```python
from build123d import *

# Parameters (mm, degrees)
SKETCH_19_R           = 3.4
MEMBER_4060_A_1_DEPTH = 800
SKETCH_14_R           = 3
CUT_EXTRUDE_1_DEPTH   = 10


with BuildPart() as part:
    # 草图19 → Member 4060-a _1 (new body)
    with BuildSketch(Plane.YZ):
        with BuildLine():
            Line((10.25, 16.5), (10.25, 12.765240679))
            Line((10.25, 12.765240679), (6.149583391, 8.63609737))
            ThreePointArc((6.149583391, 8.63609737), (5.17375715, 7.980369349), (4.020871182, 7.75))
            Line((4.020871182, 7.75), (-4.020871182, 7.75))
            ThreePointArc((-4.020871182, 7.75), (-5.17375715, 7.980369349), (-6.149583391, 8.63609737))
            Line((-6.149583391, 8.63609737), (-10.25, 12.765240679))
            Line((-10.25, 12.765240679), (-10.25, 16.5))
            ThreePointArc((-10.25, 16.5), (-9.957106781, 17.207106781), (-9.25, 17.5))
            Line((-9.25, 17.5), (-8, 17.5))
            ThreePointArc((-8, 17.5), (-7.292893219, 17.207106781), (-7, 16.5))
            Line((-7, 16.5), (-7, 15.5))
            Line((-7, 15.5), (-4.1, 15.5))
            Line((-4.1, 15.5), (-4.1, 19))
            Line((-4.1, 19), (-5.1, 19))
            Line((-5.1, 19), (-5.1, 20))
            Line((-5.1, 20), (-27.5, 20))
            ThreePointArc((-27.5, 20), (-29.267766953, 19.267766953), (-30, 17.5))
            Line((-30, 17.5), (-30, 5.1))
            Line((-30, 5.1), (-29, 5.1))
            Line((-29, 5.1), (-29, 4.1))
            Line((-29, 4.1), (-25.5, 4.1))
            Line((-25.5, 4.1), (-25.5, 7))
            Line((-25.5, 7), (-26.5, 7))
            ThreePointArc((-26.5, 7), (-27.207106781, 7.292893219), (-27.5, 8))
            Line((-27.5, 8), (-27.5, 9.25))
            ThreePointArc((-27.5, 9.25), (-27.207106781, 9.957106781), (-26.5, 10.25))
            Line((-26.5, 10.25), (-22.765240679, 10.25))
            Line((-22.765240679, 10.25), (-18.63609737, 6.149583391))
            ThreePointArc((-18.63609737, 6.149583391), (-17.980369349, 5.17375715), (-17.75, 4.020871182))
            Line((-17.75, 4.020871182), (-17.75, -4.020871182))
            ThreePointArc((-17.75, -4.020871182), (-17.980369349, -5.17375715), (-18.63609737, -6.149583391))
            Line((-18.63609737, -6.149583391), (-22.765240679, -10.25))
            Line((-22.765240679, -10.25), (-26.5, -10.25))
            ThreePointArc((-26.5, -10.25), (-27.207106781, -9.957106781), (-27.5, -9.25))
            Line((-27.5, -9.25), (-27.5, -8))
            ThreePointArc((-27.5, -8), (-27.207106781, -7.292893219), (-26.5, -7))
            Line((-26.5, -7), (-25.5, -7))
            Line((-25.5, -7), (-25.5, -4.1))
            Line((-25.5, -4.1), (-29, -4.1))
            Line((-29, -4.1), (-29, -5.1))
            Line((-29, -5.1), (-30, -5.1))
            Line((-30, -5.1), (-30, -17.5))
            ThreePointArc((-30, -17.5), (-29.267766953, -19.267766953), (-27.5, -20))
            Line((-27.5, -20), (-5.1, -20))
            Line((-5.1, -20), (-5.1, -19))
            Line((-5.1, -19), (-4.1, -19))
            Line((-4.1, -19), (-4.1, -15.5))
            Line((-4.1, -15.5), (-7, -15.5))
            Line((-7, -15.5), (-7, -16.5))
            ThreePointArc((-7, -16.5), (-7.292893219, -17.207106781), (-8, -17.5))
            Line((-8, -17.5), (-9.25, -17.5))
            ThreePointArc((-9.25, -17.5), (-9.957106781, -17.207106781), (-10.25, -16.5))
            Line((-10.25, -16.5), (-10.25, -12.765240679))
            Line((-10.25, -12.765240679), (-6.149583391, -8.63609737))
            ThreePointArc((-6.149583391, -8.63609737), (-5.17375715, -7.980369349), (-4.020871182, -7.75))
            Line((-4.020871182, -7.75), (4.020871182, -7.75))
            ThreePointArc((4.020871182, -7.75), (5.17375715, -7.980369349), (6.149583391, -8.63609737))
            Line((6.149583391, -8.63609737), (10.25, -12.765240679))
            Line((10.25, -12.765240679), (10.25, -16.5))
            ThreePointArc((10.25, -16.5), (9.957106781, -17.207106781), (9.25, -17.5))
            Line((9.25, -17.5), (8, -17.5))
            ThreePointArc((8, -17.5), (7.292893219, -17.207106781), (7, -16.5))
            Line((7, -16.5), (7, -15.5))
            Line((7, -15.5), (4.1, -15.5))
            Line((4.1, -15.5), (4.1, -19))
            Line((4.1, -19), (5.1, -19))
            Line((5.1, -19), (5.1, -20))
            Line((5.1, -20), (27.5, -20))
            ThreePointArc((27.5, -20), (29.267766953, -19.267766953), (30, -17.5))
            Line((30, -17.5), (30, -5.1))
            Line((30, -5.1), (29, -5.1))
            Line((29, -5.1), (29, -4.1))
            Line((29, -4.1), (25.5, -4.1))
            Line((25.5, -4.1), (25.5, -7))
            Line((25.5, -7), (26.5, -7))
            ThreePointArc((26.5, -7), (27.207106781, -7.292893219), (27.5, -8))
            Line((27.5, -8), (27.5, -9.25))
            ThreePointArc((27.5, -9.25), (27.207106781, -9.957106781), (26.5, -10.25))
            Line((26.5, -10.25), (22.765240679, -10.25))
            Line((22.765240679, -10.25), (18.63609737, -6.149583391))
            ThreePointArc((18.63609737, -6.149583391), (17.980369349, -5.17375715), (17.75, -4.020871182))
            Line((17.75, -4.020871182), (17.75, 4.020871182))
            ThreePointArc((17.75, 4.020871182), (17.980369349, 5.17375715), (18.63609737, 6.149583391))
            Line((18.63609737, 6.149583391), (22.765240679, 10.25))
            Line((22.765240679, 10.25), (26.5, 10.25))
            ThreePointArc((26.5, 10.25), (27.207106781, 9.957106781), (27.5, 9.25))
            Line((27.5, 9.25), (27.5, 8))
            ThreePointArc((27.5, 8), (27.207106781, 7.292893219), (26.5, 7))
            Line((26.5, 7), (25.5, 7))
            Line((25.5, 7), (25.5, 4.1))
            Line((25.5, 4.1), (29, 4.1))
            Line((29, 4.1), (29, 5.1))
            Line((29, 5.1), (30, 5.1))
            Line((30, 5.1), (30, 17.5))
            ThreePointArc((30, 17.5), (29.267766953, 19.267766953), (27.5, 20))
            Line((27.5, 20), (5.1, 20))
            Line((5.1, 20), (5.1, 19))
            Line((5.1, 19), (4.1, 19))
            Line((4.1, 19), (4.1, 15.5))
            Line((4.1, 15.5), (7, 15.5))
            Line((7, 15.5), (7, 16.5))
            ThreePointArc((7, 16.5), (7.292893219, 17.207106781), (8, 17.5))
            Line((8, 17.5), (9.25, 17.5))
            ThreePointArc((9.25, 17.5), (9.957106781, 17.207106781), (10.25, 16.5))
        make_face()
        Circle(SKETCH_19_R, mode=Mode.SUBTRACT)
        Polygon((27.5, -12.75), (27.5, -17.5), (12.75, -17.5), (12.75, -9.5), (18.462046185, -9.5), (21.734815036, -12.75), align=None, mode=Mode.SUBTRACT)
        Polygon((5.9, 5.25), (10.25, 5.25), (10.25, 7), (15.25, 7), (15.25, -7), (10.25, -7), (10.25, -5.25), (5.9, -5.25), align=None, mode=Mode.SUBTRACT)
        Polygon((-27.5, 12.75), (-27.5, 17.5), (-12.75, 17.5), (-12.75, 9.5), (-18.462046185, 9.5), (-21.734815036, 12.75), align=None, mode=Mode.SUBTRACT)
        Polygon((27.5, 17.5), (27.5, 12.75), (21.734815036, 12.75), (18.462046185, 9.5), (12.75, 9.5), (12.75, 17.5), align=None, mode=Mode.SUBTRACT)
        Polygon((-10.25, 7), (-10.25, 5.25), (-5.9, 5.25), (-5.9, -5.25), (-10.25, -5.25), (-10.25, -7), (-15.25, -7), (-15.25, 7), align=None, mode=Mode.SUBTRACT)
        Polygon((-27.5, -17.5), (-27.5, -12.75), (-21.734815036, -12.75), (-18.462046185, -9.5), (-12.75, -9.5), (-12.75, -17.5), align=None, mode=Mode.SUBTRACT)
    extrude(amount=MEMBER_4060_A_1_DEPTH)

    # 草图14 → 切除-拉伸1 (cut)
    with BuildSketch(Plane(origin=(0, -12.75, 0), x_dir=(-1, 0, 0), z_dir=(0, -1, 0))):
        with Locations(Location((-785, 0, 0), (0, 0, 90))):
            Circle(SKETCH_14_R)
    extrude(amount=-CUT_EXTRUDE_1_DEPTH, mode=Mode.SUBTRACT)


solid = part.part
```
Geometry: final body of the model. Coordinates: model frame, mm. A direction names the side the tool comes from. Coordinates: 2 decimals unless noted, no trailing zeros.
Item 1: Material intervals for line 1 along Y through (x, z) = (672, 13); line 2 along Y through (x, z) = (382, -4); line 3 along Z through (x, y) = (785, -5.05), sorted ascending.
Answer:
line 1: y = -30 to -27.5, -12.75 to -10.25, 10.25 to 12.75, 27.5 to 30
line 2: y = -17.75 to -15.25, -5.9 to 5.9, 15.25 to 17.75
line 3: z = -19 to -15.5, -7.93 to -3, 3 to 7.93, 15.5 to 19
Item 2: Contact query for flat-ended pins moving along their axis: P1, Ø0.8, axis at x = 552.5, z = 19.5, coming from the -Y side; P2, Ø2.5, axis at x = 302.5, y = 0.5, coming from the +Z side; P3, Ø6, axis at y = -22, z = -4.5, coming from the +X side. Output: stop coordinate, or through.
Answer:
P1: stops at y = -29.42
P2: stops at z = 7.75
P3: passes through
Item 3: Access query for faces 1 (the face through (394, 16, -20)), 2 (the face through (394, -20, -17.5)). Directions: +Z, -Z, +X, -X, +Y, -Y. A direction counts if a zero-diameter tool reaches every point of the face in a straight line with its end or side. Return the directions, or none.
Answer:
face 1: -Z, +X, -X, +Y, -Y
face 2: +X, -X
Item 4: Section query A-A (x = 533.5). State how many separate pieces and enclosed holes the cut face has, then the cut area to 3 significant figures.
Answer:
separate pieces: 1
enclosed holes: 7
area: 1,010 mm2
Item 5: Draft query along Y for faces 3 (the face through (394, 15.25, 0)), 4 (the face through (394, -16, 20)), 5 (the face through (394, -30, 11)). Return one class per face: released by +Y, released by -Y, zero draft, split by the parting line, or undercut.
Answer:
face 3: undercut
face 4: zero draft
face 5: released by -Y
